The model under review builds one solid part; all positions refer to its coordinate system, in mm. A direction names the side the tool comes from. Coordinates: 2 decimals unless noted, no trailing zeros. Write each loop counter-clockwise with the first axis right and the second up, starting at its lowest first coordinate (ties: lowest second). Pieces come first, ordered by that corner, then holes. Notation, with made-up numbers: (68, 74) - (92, 74) arc R13 ccw to (92, 87) - close; hole circle Ø7 at (58.25, 60.5). An arc over 180 degrees is marked (long way). Put each result on its own line as item: value. Start each with the question number.
Item 1: For pin 1 (1.5 mm diameter, centred on y = 0.5, z = 49, fed in from -X); pin 2 (8 mm diameter, centred on x = -1, y = -2, fed in from -Z); pin 3 (2.5 mm diameter, centred on x = 0, z = 57, fed in from +Y); pin 4 (1.2 mm diameter, centred on y = 12, z = 51, fed in from -X), all flat-tipped, find the tip position at first contact; note any pin that passes through.
Item 2: Consider section B-B on z = 75.5. Give the boundary of the cut face in (x, y), then the cut area to 3 significant figures.
Item 3: Consider section C-C on x = 10. Give the boundary of the cut face in (y, z) (3 decimals).
Item 4: Mouldability with a two-part tool opening along X and no side actions: class faces 1 (the face through (0.54, -12.69, 48.33)), 2 (the face through (-12.3, -1.9, 86.106)), 3 (the face through (0, 7, 80.2)) as pulls with the +X half, pulls with the -X half, needs draft (parallel to the pull), parting line crosses it, or undercut.
Item 5: To check wall thickness, follow L1, parallel to Y at x = 0, z = 49; L2, parallel to Z at x = -1, y = -13.5; L3, parallel to Y at x = 0, z = 85. State the ranges of each line that lie inside material, in increasing order. Write a range as [from, to].
Item 6: Machinability: for faces 4 (the face through (-1.72, -7.75, 84.22)), 5 (the face through (1.72, -7.75, 3.91)), 6 (the face through (0.51, -12.18, 85.53)), 7 (the face through (0, 11.112, 50)), which of the approach directions +Z, -Z, +X, -X, +Y, -Y give a long, thin tool a straight path to every point of the face, cutting with its end or side? Answer none if there is none.
Autodesk Inventor part; units mm, degrees
ref_plane "Work Plane5" through (0, 0, 84.963) normal (0, 0, 1) x (1, 0, 0)
ref_plane "Work Plane6" through (0, 0, 15.113) normal (0, 0, -1) x (-1, 0, 0)
ref_plane "Work Plane10" through (0, 0, 29.464) normal (0, 0, -1) x (-1, 0, 0)
sketch "Sketch1" plane through (0, 0, 0) normal (0, 0, 1) x (1, 0, 0)
  circle A0 centre (0, 0) radius 12.7
  circle A1 centre (0, 0) radius 6.35
  line L0 (-1.5875, 14.2875) -> (1.5875, 14.2875)
  line L1 (1.5875, 14.2875) -> (1.5875, 11.1125)
  line L2 (1.5875, 11.1125) -> (-1.5875, 11.1125)
  line L3 (-1.5875, 11.1125) -> (-1.5875, 14.2875)
  dimension "d0" = 25.4
  dimension "d4" = 12.7
  dimension "d50" = 3.175
  dimension "d51" = 3.175
  dimension "d52" = 1.5875
  dimension "d53" = 14.2875
extrude "Extrusion4" add sketch "Sketch1" along normal blind 88.138 contours A0 L3 L2 L1 | L1 L2 L3 A0
ref_plane "Work Plane5" through (0, 0, 84.963) normal (0, 0, 1) x (1, 0, 0)
sketch "Sketch6" plane through (0, 0, 84.963) normal (0, 0, 1) x (1, 0, 0)
  circle A0 centre (0, 0) radius 12.192
  circle A1 centre (0, 0) radius 12.7
  dimension "d24" = 24.384
extrude "Extrusion8" cut sketch "Sketch6" along normal blind 1.143
ref_plane "Work Plane6" through (0, 0, 15.113) normal (0, 0, -1) x (-1, 0, 0)
ref_plane "Work Plane9" through (0, 0, 43.3324) normal (0, 0, -1) x (-1, 0, 0)
ref_plane "Work Plane10" through (0, 0, 29.464) normal (0, 0, -1) x (-1, 0, 0)
extrude "Extrusion16" cut sketch "Sketch1" along normal through all contours L1 L2 L3 A0 | A0 L3 L0 L1 picked at (0.1768, 11.638)
sketch "Sketch14" plane through (0, 0, 88.138) normal (0, 0, 1) x (1, 0, 0)
  circle A0 centre (0, 0) radius 6.35
  circle A1 centre (0, 0) radius 7.9375
  dimension "d56" = 15.875
extrude "Extrusion17" cut sketch "Sketch14" against normal blind 7.9375
sketch "Sketch15" plane through (0, 0, 0) normal (0, 0, -1) x (-1, 0, 0)
  circle A0 centre (0, 0) radius 6.35
  circle A1 centre (0, 0) radius 7.9375
  dimension "d59" = 15.875
extrude "Extrusion18" cut sketch "Sketch15" against normal blind 7.9375
ref_plane "Work Plane13" through (0, 0, 6.35) normal (0, 0, -1) x (-1, 0, 0)
sketch "Sketch16" plane through (0, 0, 6.35) normal (0, 0, -1) x (-1, 0, 0)
  arc A0 (-1.5875, 12.6004) -> (1.5875, 12.6004) centre (0, 0) ccw
  line L0 (-1.5875, 12.6004) -> (-1.5875, 11.1125)
  line L1 (-1.5875, 11.1125) -> (1.5875, 11.1125)
  line L2 (1.5875, 11.1125) -> (1.5875, 12.6004)
  circle A1 centre (0, 0) radius 15.875
  circle A2 centre (0, 0) radius 14.2875
  dimension "d63" = 31.75
  dimension "d68" = 28.575
extrude "Extrusion19" add sketch "Sketch16" against normal blind 3.175 contours A1 | A2
sketch "Sketch17" plane through (0, 0, 0) normal (0, 0, -1) x (-1, 0, 0)
  line L0 (-1.5875, 11.1125) -> (-1.5875, 12.6004)
  arc A0 (-1.5875, 12.6004) -> (1.5875, 12.6004) centre (0, 0) ccw
  line L1 (1.5875, 12.6004) -> (1.5875, 11.1125)
  line L2 (1.5875, 11.1125) -> (-1.5875, 11.1125)
  arc A1 (1.5875, 12.6004) -> (-1.5875, 12.6004) centre (0, 0) ccw
extrude "Extrusion20" add sketch "Sketch17" against normal blind 6.35 contours L0 A1 L1 L2
extrude "Extrusion21" add sketch "Sketch16" against normal blind 6.35 contours A2
equation "\"d51\" = d50"
properties part number "turn shaft"
Report:
1. pin 1: x = -12.7
1. pin 2: through
1. pin 3: y = 11.11
1. pin 4: x = -5.6
2. outline: (-1.59, 11.11) - (-1.59, 12.6) arc R12.7 ccw (long way) to (1.59, 12.6) - (1.59, 11.11) - close; hole circle Ø12.7 at (0, 0)
2. area: 375 mm²
3. outline: (-12.329, 6.35) - (-7.829, 6.35) - (-7.829, 0) - (7.829, 0) - (7.829, 6.35) - (12.329, 6.35) - (12.329, 9.525) - (10.205, 9.525) - (10.205, 12.7) - (7.829, 12.7) - (7.829, 84.963) - (6.975, 84.963) - (6.975, 86.106) - (7.829, 86.106) - (7.829, 88.138) - (-7.829, 88.138) - (-7.829, 86.106) - (-6.975, 86.106) - (-6.975, 84.963) - (-7.829, 84.963) - (-7.829, 12.7) - (-10.205, 12.7) - (-10.205, 9.525) - (-12.329, 9.525) - close
4. face 1: parting line crosses it
4. face 2: needs draft
4. face 3: undercut
5. L1: [-12.7, -6.35], [6.35, 11.11]
5. L2: [6.35, 12.7]
5. L3: [-12.19, -7.94], [7.94, 11.11]
6. face 4: +Z
6. face 5: -Z
6. face 6: none
6. face 7: +Z, +Y
